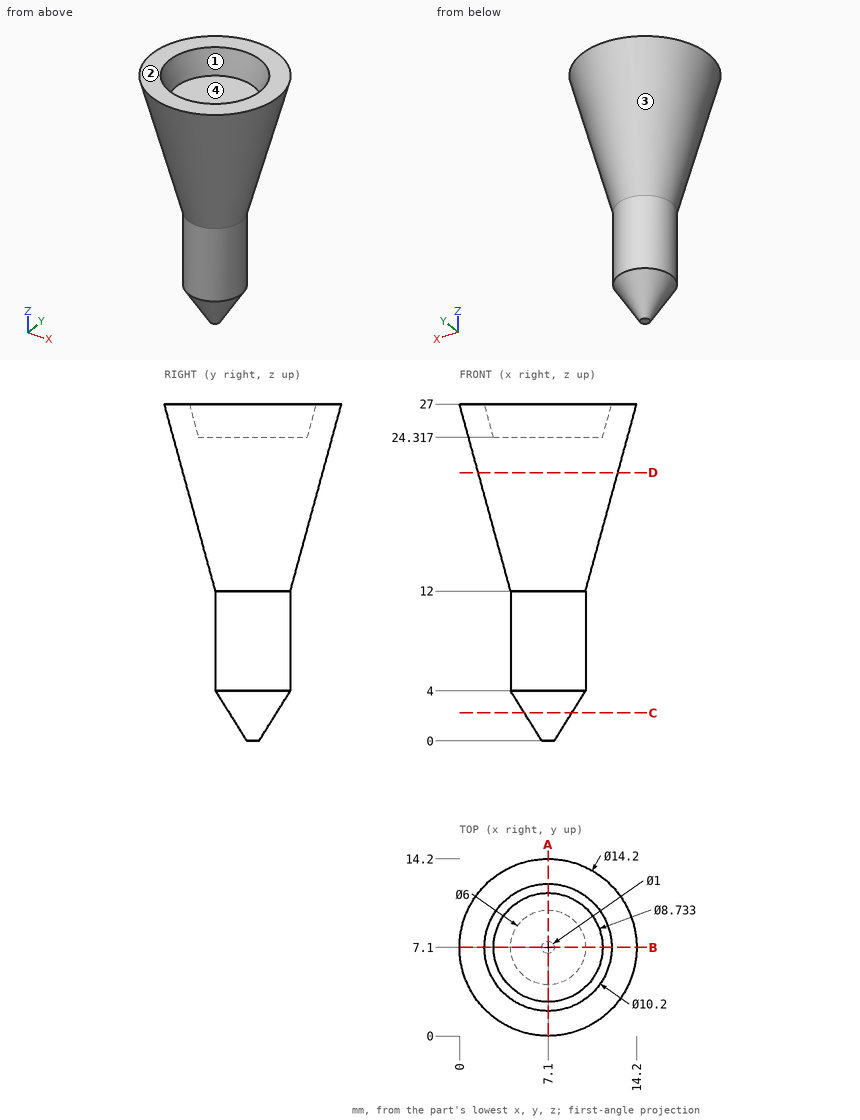
Geometry: see drawing. Coordinates: mm, zero at the bounding-box minimum. Give positions to 0.01 mm unless a question says otherwise; leave off trailing zeros. Order: outer loops, then holes, each group sorted by start corner. A loop starts at its lowest first (then second) coordinate and runs counter-clockwise, first axis right, second up. Notation, with made-up numbers: (-17.75, 29.5) -> (3.25, 29.5) arc R25 ccw to (3.25, 45.5) -> close; hole circle Ø5 at (4.5, -30). An arc over 180 degrees is marked (long way). Write each question's results on one line, items separated by ' | '.
1) Cut plane C-C (z = 2.25). Output: boundary loops of the cut face in (x, y).
Geometry says:
outline: circle Ø3.81 at (7.1, 7.1)
2) Cut plane A-A (x = 7.1). Output: boundary loops of the cut face in (y, z), and give its area (3 significant figures).
Geometry says:
outline: (0, 27) -> (4.1, 12) -> (4.1, 4) -> (6.6, 0) -> (7.6, 0) -> (10.1, 4) -> (10.1, 12) -> (14.2, 27) -> (12.2, 27) -> (11.47, 24.32) -> (2.73, 24.32) -> (2, 27) -> close | area: 188 mm²
3) Draft query along X for the marked faces 1, 2, 3 and 4. Return one class per face: released by +X, released by -X, zero draft, split by the parting line, or undercut.
Geometry says:
face 1: undercut | face 2: zero draft | face 3: split by the parting line | face 4: undercut
4) First-contact query: pin 1 Ø6 at (x, y) = (7, 6.5) entering from +Z; pin 2 Ø4 at (y, z) = (11, 16.5) entering from +X; pin 3 Ø5 at (x, z) = (5, 4) entering from -Y. Flat tips, straight axial feed; report the tip coordinate or a pass-through.
Geometry says:
pin 1: stops at z = 24.32 | pin 2: stops at x = 11.05 | pin 3: stops at y = 4.1
5) Cut plane D-D (z = 21.5). Output: boundary loops of the cut face in (x, y).
Geometry says:
outline: circle Ø11.19 at (7.1, 7.1)
6) Line query: line 1 along Y through (x, z) = (4, 25) (1 decimal); line 2 along X through (y, z) = (9.5, 25); line 3 along Y through (x, z) = (8, 10). Output: solid intervals per line, ascending.
Geometry says:
line 1: y = 1.3 to 3.8, 10.4 to 12.9 | line 2: x = 1 to 3.23, 10.97 to 13.2 | line 3: y = 4.24 to 9.96
